```python
from build123d import *

# Parameters (mm, degrees)
F0_R     = 12.5
F1_DEPTH = 21
F2_W     = 11
F2_H     = 20
F4_W     = 67.492016
F4_H     = 6.775262
F5_DEPTH = 48.001


with BuildPart() as f1:
    # F0 (on Top) → F1 (new body)
    with BuildSketch(Plane.XY):
        with BuildLine():
            ThreePointArc((0, 17.5), (5.125631, 5.125631), (17.5, 0))
            Line((17.5, 0), (62, 0))
            ThreePointArc((62, 0), (65.535534, 1.464466), (67, 5))
            Line((67, 5), (67, 43))
            ThreePointArc((67, 43), (65.535534, 46.535534), (62, 48))
            Line((62, 48), (5, 48))
            ThreePointArc((5, 48), (1.464466, 46.535534), (0, 43))
            Line((0, 43), (0, 17.5))
        make_face()
        with Locations((17.5, 17.5)):
            Circle(F0_R, mode=Mode.SUBTRACT)
    extrude(amount=F1_DEPTH)

    # F2 (on face) → F3 (revolve, cut)
    with BuildSketch(Plane.XY.offset(21)):
        with Locations((40.5, 15)):
            Rectangle(F2_W, F2_H)
        with Locations((56.5, 15)):
            Rectangle(F2_W, F2_H)
    revolve(axis=Axis((40.5, 25, 21), (1, 0, 0)), mode=Mode.SUBTRACT)

    # F4 (on face) → F5 (cut, through all)
    with BuildSketch(Plane.XZ):
        with Locations((33.746008, 18.387631)):
            Rectangle(F4_W, F4_H)
    extrude(amount=-F5_DEPTH, mode=Mode.SUBTRACT)


solid = f1.part
```
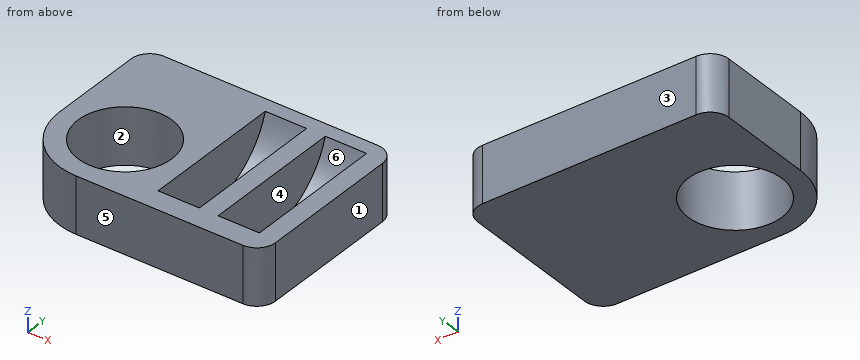
The listing builds one solid part. Answer for the finished solid, in the listing's coordinates (mm). Face numbers are marked on the shaded views. A direction names the side the tool comes from. Round coordinates to 2 decimals unless told otherwise and drop trailing zeros. Write each loop counter-clockwise with the first axis right and the second up, starting at its lowest first coordinate (ties: lowest second). Pieces come first, ordered by that corner, then holes. Notation, with made-up numbers: (-27.5, 9) -> (31.5, 9) arc R22 ccw to (31.5, 28) -> close; hole circle Ø8 at (-39.75, -0.75). An arc over 180 degrees is marked (long way). Use CSV: the item, a comma, the result in double quotes. Start each with the question number.
(1) Section B-B on x = 9 is taken. Give the vertices of the cut face in (y, z), then the cut area to 3 significant figures.
(2) Consider L1, parallel to X at y = 17.5, z = 10.5; L2, parallel to X at y = 41, z = 10.5; L3, parallel to Y at x = 17.5, z = 11. Determine where each line is inside the solid, lowest interval first. Write a range as from..to.
(3) Section D-D on x = 19 is taken. Give the vertices of the cut face in (y, z), then the cut area to 3 significant figures.
(4) This flat-tipped pin is pushed along its axis until it touches: pin 1 (12 mm diameter, centred on x = 23.5, y = 27, fed in from +Z). Where does it stop, or does it pass through?
(5) Section C-C on z = 8 is taken. Give the vertices of the cut face in (x, y), then the cut area to 3 significant figures.
(6) Section A-A on y = 25 is taken. Give the vertices of the cut face in (x, z).
(7) The mould has two halves that part along Y. Classify the marked faces 1, 2, 3 and 4: released by +Y, released by -Y, zero draft, split by the parting line, or undercut.
(8) Which of the six approach directions +Z, -Z, +X, -X, +Y, -Y give full straight-line access (tool end or side, diameter ignored) to the marked faces 5 and 6?
A:
1,outline,"(2.2, 0) -> (8.33, 0) -> (8.33, 15) -> (2.2, 15) -> close; (26.67, 0) -> (48, 0) -> (48, 15) -> (26.67, 15) -> close"
1,area,"412 mm²"
2,L1,"x = 0..5, 30..35, 46..51, 62..67"
2,L2,"x = 0..35, 46..51, 62..67"
2,L3,"y = 0..5, 30..48"
3,outline,"(0, 0) -> (5.09, 0) -> (5.09, 15) -> (0, 15) -> close; (29.91, 0) -> (48, 0) -> (48, 15) -> (29.91, 15) -> close"
3,area,"348 mm²"
4,pin 1,"stops at z = 15"
5,outline,"(0, 17.5) arc R17.5 ccw to (17.5, 0) -> (62, 0) arc R5 ccw to (67, 5) -> (67, 43) arc R5 ccw to (62, 48) -> (5, 48) arc R5 ccw to (0, 43) -> close; hole circle Ø25 at (17.5, 17.5); hole (35, 9.8) -> (46, 9.8) -> (46, 40.2) -> (35, 40.2) -> close; hole (51, 9.8) -> (62, 9.8) -> (62, 40.2) -> (51, 40.2) -> close"
5,area,"1,970 mm²"
6,outline,"(0, 0) -> (7.5, 0) -> (7.5, 15) -> (0, 15) -> close; (27.5, 0) -> (67, 0) -> (67, 15) -> (62, 15) -> (62, 1) -> (51, 1) -> (51, 15) -> (46, 15) -> (46, 1) -> (35, 1) -> (35, 15) -> (27.5, 15) -> close"
7,face 1,"zero draft"
7,face 2,"undercut"
7,face 3,"released by +Y"
7,face 4,"undercut"
8,face 5,"+Z, -Z, +X, -X, -Y"
8,face 6,"+Z"
